Input: part model. Units: mm. Frame: model coordinates. Face numbers are marked on the shaded views. A direction names the side the tool comes from. Coordinates: 2 decimals unless noted, no trailing zeros. Order: outer loops, then holes, each group sorted by start corner. A loop starts at its lowest first (then second) coordinate and runs counter-clockwise, first axis right, second up. Notation, with made-up numbers: (23, -27.75) -> (81, -27.75) arc R12 cw to (81, -15.75) -> close; hole circle Ø8 at (-4, -5.5). An arc over 180 degrees is marked (long way). Write each question's results on one line, items separated by ' | '.
```python
from build123d import *

# Parameters (mm, degrees)
SKETCH1_W           = 120
SKETCH1_H           = 40
BOSS_EXTRUDE1_DEPTH = 30
CUT_EXTRUDE1_DEPTH  = 60
CUT_EXTRUDE2_DEPTH  = 60
SKETCH4_W           = 30
SKETCH4_H           = 30
BOSS_EXTRUDE2_DEPTH = 10
SKETCH5_R           = 10
CUT_EXTRUDE3_DEPTH  = 1
SKETCH7_R           = 6
CUT_EXTRUDE5_DEPTH  = 55
SKETCH6_W           = 10
SKETCH6_H           = 10
CUT_EXTRUDE4_DEPTH  = 10
CHAMFER1_SIZE       = 2
SKETCH8_R           = 6
CUT_EXTRUDE6_DEPTH  = 55


with BuildPart() as part:
    # Sketch1 → Boss-Extrude1 (new body)
    with BuildSketch(Plane.XY):
        Rectangle(SKETCH1_W, SKETCH1_H)
    extrude(amount=BOSS_EXTRUDE1_DEPTH)

    # Sketch2 → Cut-Extrude1 (cut)
    with BuildSketch(Plane(origin=(60, 0, 0), x_dir=(0, 0, -1), z_dir=(1, 0, 0))):
        Polygon((-30, 16), (-19.782067596, 16), (-17, 16), (-17, 10), (-19.5, 10), (-19.5, -16), (-30, -16), align=None)
    extrude(amount=-CUT_EXTRUDE1_DEPTH, mode=Mode.SUBTRACT)

    # Sketch3 → Cut-Extrude2 (cut)
    with BuildSketch(Plane.ZY.offset(60)):
        Polygon((30, 16), (19.5, 16), (19.5, -10), (17, -10), (17, -16), (18.436994707, -16), (30, -16), align=None)
    extrude(amount=-CUT_EXTRUDE2_DEPTH, mode=Mode.SUBTRACT)

    # Sketch4 → Boss-Extrude2 (add)
    with BuildSketch(Plane(origin=(0, 0, 0), x_dir=(-1, 0, 0), z_dir=(0, 0, -1))):
        Rectangle(SKETCH4_W, SKETCH4_H)
    extrude(amount=BOSS_EXTRUDE2_DEPTH)

    # Sketch5 → Cut-Extrude3 (cut)
    with BuildSketch(Plane(origin=(60, 0, 0), x_dir=(0, 0, -1), z_dir=(1, 0, 0))):
        with Locations((-12, 12)):
            Circle(SKETCH5_R)
        with Locations((-12, -12)):
            Circle(SKETCH5_R)
    cut_extrude3 = extrude(amount=-CUT_EXTRUDE3_DEPTH, mode=Mode.SUBTRACT)

    # Sketch7 → Cut-Extrude5 (cut)
    with BuildSketch(Plane(origin=(59, 0, 0), x_dir=(0, 0, -1), z_dir=(1, 0, 0))):
        with Locations((-12, -12)):
            Circle(SKETCH7_R)
    extrude(amount=-CUT_EXTRUDE5_DEPTH, mode=Mode.SUBTRACT)

    # Mirror1: Cut-Extrude3 across plane
    add(cut_extrude3.mirror(Plane(origin=(0, 0, 0), x_dir=(0, 0, 1), z_dir=(1, 0, 0))), mode=Mode.SUBTRACT)

    # Sketch6 → Cut-Extrude4 (cut)
    with BuildSketch(Plane.XY.offset(19.5)):
        Rectangle(SKETCH6_W, SKETCH6_H)
    extrude(amount=-CUT_EXTRUDE4_DEPTH, mode=Mode.SUBTRACT)

    # Chamfer1
    chamfer1_edges = [part.edges().sort_by_distance(p)[0] for p in [
        (0, -16, 30),
        (0, 16, 30),
    ]]
    chamfer(chamfer1_edges, length=CHAMFER1_SIZE)

    # Sketch8 → Cut-Extrude6 (cut)
    with BuildSketch(Plane.ZY.offset(59)):
        with Locations((12, 12)):
            Circle(SKETCH8_R)
    extrude(amount=-CUT_EXTRUDE6_DEPTH, mode=Mode.SUBTRACT)


solid = part.part
```
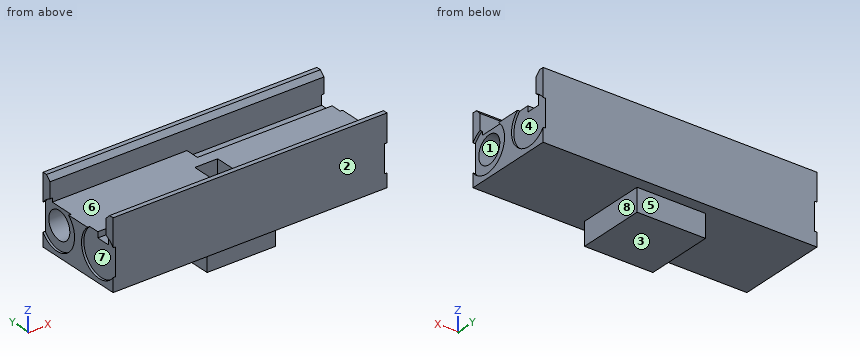
(1) Cut plane A-A, the plane z = 12. Return loops of the section in (x, y).
Return value:
outline: (-60, -2) -> (-59, -2) -> (-59, -20) -> (59, -20) -> (59, -18) -> (4, -18) -> (4, -6) -> (59, -6) -> (59, -2) -> (60, -2) -> (60, 2) -> (59, 2) -> (59, 20) -> (-59, 20) -> (-59, 18) -> (-4, 18) -> (-4, 6) -> (-59, 6) -> (-59, 2) -> (-60, 2) -> close; hole (-5, -5) -> (5, -5) -> (5, 5) -> (-5, 5) -> close
(2) Reachability of the marked faces 5, 6, 7 and 8 from +Z, -Z, +X, -X, +Y, -Y: full face, straight path, thin tool, end or side. Return the list, or none.
Return value:
face 5: -Z, +X, -X, +Y | face 6: +Z, +X, -X | face 7: -X | face 8: -Z, +X, +Y, -Y
(3) Line query: line 1 along Y through (x, z) = (33.5, 23); line 2 along Z through (x, y) = (-33.5, -8); line 3 along Z through (x, y) = (-59.3, 12). Output: solid intervals per line, ascending. Write a range as from..to.
Return value:
line 1: -20..-16, 16..20 | line 2: 0..19.5 | line 3: 0..2
(4) Cut plane B-B, the plane x = 38. Return loops of the section in (y, z).
Return value:
outline: (-20, 0) -> (20, 0) -> (20, 30) -> (18, 30) -> (16, 28) -> (16, 17) -> (10, 17) -> (10, 19.5) -> (-16, 19.5) -> (-16, 28) -> (-18, 30) -> (-20, 30) -> close; hole circle Ø12 at (-12, 12)
(5) Mould query, pull axis Y, two halves, no side actions, for the marked faces 1, 2, 3 and 4. Classes: +Y half, -Y half, draft (parallel to the pull), parting line (faces both ways), or undercut.
Return value:
face 1: undercut | face 2: -Y half | face 3: draft | face 4: undercut
(6) Cut plane D-D, the plane x = 9.5. Return loops of the section in (y, z).
Return value:
outline: (-20, 0) -> (-15, 0) -> (-15, -10) -> (15, -10) -> (15, 0) -> (20, 0) -> (20, 30) -> (18, 30) -> (16, 28) -> (16, 17) -> (10, 17) -> (10, 19.5) -> (-16, 19.5) -> (-16, 28) -> (-18, 30) -> (-20, 30) -> close; hole circle Ø12 at (-12, 12)
(7) Pin query (flat end, axial travel): P1, Ø6, axis at x = 34.5, y = 15.5, coming from the -Z side; P2, Ø6.5, axis at x = -26, y = -12, coming from the +Z side; P3, Ø2, axis at y = 13, z = 18.5, coming from the +X side. Return the tip coordinate at first contact, or that it passes through.
Return value:
P1: z = 0 | P2: z = 19.5 | P3: x = 0
(8) Cut plane C-C, the plane y = 0.5. Return loops of the section in (x, z), plus the area to 3 significant figures.
Return value:
outline: (-60, 0) -> (-15, 0) -> (-15, -10) -> (15, -10) -> (15, 0) -> (60, 0) -> (60, 19.5) -> (5, 19.5) -> (5, 9.5) -> (-5, 9.5) -> (-5, 19.5) -> (-60, 19.5) -> close | area: 2,540 mm2
